```python
from build123d import *

# Parameters (mm, degrees)
SKETCH2_R               = 1.5
BOSS_EXTRUDE1_DEPTH     = 8
CUT_EXTRUDE1_DEPTH      = 18
CUT_EXTRUDE1_DEPTH_BACK = 18
CUT_EXTRUDE2_DEPTH      = 5
CUT_EXTRUDE3_DEPTH      = 1.5


with BuildPart() as part:
    # Sketch2 → Boss-Extrude1 (new body)
    with BuildSketch(Plane.XY):
        with BuildLine():
            Line((-3.5, 5), (3.5, 5))
            ThreePointArc((3.5, 5), (8.5, 0), (3.5, -5))
            Line((3.5, -5), (-3.5, -5))
            ThreePointArc((-3.5, -5), (-8.5, 0), (-3.5, 5))
        make_face()
        with Locations((-3.5, 0)):
            Circle(SKETCH2_R, mode=Mode.SUBTRACT)
    extrude(amount=BOSS_EXTRUDE1_DEPTH)

    # Sketch3 → Cut-Extrude1 (cut, two sides)
    with BuildSketch(Plane(origin=(0, 0, 0), x_dir=(0, 0, -1), z_dir=(1, 0, 0))) as cut_extrude1_sk:
        Polygon((-8, -2), (-4.5, -2), (-4.5, 2), (-6, 2), (-6, 5), (-8, 5), align=None)
    extrude(amount=CUT_EXTRUDE1_DEPTH, mode=Mode.SUBTRACT)
    extrude(cut_extrude1_sk.sketch, amount=-CUT_EXTRUDE1_DEPTH_BACK, mode=Mode.SUBTRACT)

    # Sketch4 → Cut-Extrude2 (cut)
    with BuildSketch(Plane.XY.offset(8)):
        with BuildLine():
            Line((-1.263932023, -2), (2.736067977, 5))
            Line((2.736067977, 5), (-10.787192153, 5))
            Line((-10.787192153, 5), (-10.787192153, -2))
            Line((-10.787192153, -2), (-5.736067977, -2))
            ThreePointArc((-5.736067977, -2), (-3.5, -3), (-1.263932023, -2))
        make_face()
    extrude(amount=-CUT_EXTRUDE2_DEPTH, mode=Mode.SUBTRACT)

    # Sketch5 → Cut-Extrude3 (cut)
    with BuildSketch(Plane.XY.offset(3)):
        Polygon((1.021782263, 2), (2.736067977, 5), (-9.199414094, 5), (-9.199414094, 2), align=None)
    extrude(amount=-CUT_EXTRUDE3_DEPTH, mode=Mode.SUBTRACT)


solid = part.part
```
Here's how the part is built. I have some questions about the finished solid (model axes, mm). A direction names the side the tool comes from. Coordinates: 2 decimals unless noted, no trailing zeros. Loops run counter-clockwise (first coordinate to the right, second up) from the corner with the lowest first, then second, coordinate; pieces in that order, holes last. Notation, with made-up numbers: (67.5, -2) -> (120.5, -2) arc R21 ccw to (120.5, 18) -> close; hole circle Ø6 at (63.25, -18.5). An arc over 180 degrees is marked (long way). Return JSON: item names as keys, results as strings.
1) For faces 4 (the face through (-3, 4, 1.5)), 5 (the face through (-3.5, -3, 5.5)), 6 (the face through (5, 3, 6)), 7 (the face through (5, 0, 4.5)), which set-ups out of +Z, -Z, +X, -X, +Y, -Y let a thin tool reach every point of the face, with its end or its side?
Results below:
{"face 4": "+Z, -X, +Y", "face 5": "+Z, +Y", "face 6": "+Z, +X, -X, +Y", "face 7": "+Z, +X, -X"}
2) If we section it at D-D, the plane z = 6.75: Write out the boundary of the cut face in (x, y).
Results below:
{"outline": "(-8.08, -2) arc R5 ccw to (-3.5, -5) -> (3.5, -5) arc R5 ccw to (8.08, -2) -> (-1.26, -2) arc R3 cw to (-5.74, -2) -> close"}
3) Will these pins go through, and if not, where does the flat tip stop? pin 1 (1.2 mm diameter, centred on x = -7, z = 5.5, fed in from +Y); pin 2 (4 mm diameter, centred on x = -3.5, y = 0, fed in from +Z); pin 3 (2 mm diameter, centred on x = 4, y = 0, fed in from +Z).
Results below:
{"pin 1": "y = -2", "pin 2": "z = 3", "pin 3": "z = 4.5"}
4) Thinking about a two-plate mould opening in X: for faces 1 (the face through (0, -5, 4)), 2 (the face through (-5, 1, 3)), 3 (the face through (-7.259, -3.297, 3.055)), which applies, +X half, -X half, draft (parallel to the pull), parting line (faces both ways), or undercut?
Results below:
{"face 1": "draft", "face 2": "undercut", "face 3": "-X half"}
5) If we section it at A-A, the plane z = 3.25: Write out the boundary of the cut face in (x, y).
Results below:
{"outline": "(-8.08, -2) arc R5 ccw to (-3.5, -5) -> (3.5, -5) arc R5 ccw to (3.5, 5) -> (2.74, 5) -> (-1.26, -2) arc R3 cw to (-5.74, -2) -> close"}
6) If we section it at B-B, the plane y = 0: Write out the boundary of the cut face in (x, z).
Results below:
{"outline": "(-8.5, 0) -> (-5, 0) -> (-5, 3) -> (-8.5, 3) -> close; (-2, 0) -> (8.5, 0) -> (8.5, 4.5) -> (-0.12, 4.5) -> (-0.12, 3) -> (-2, 3) -> close"}
7) If we section it at C-C, the plane x = 7.5: Write out the boundary of the cut face in (y, z), then the cut area to 3 significant figures.
Results below:
{"outline": "(-3, 0) -> (3, 0) -> (3, 6) -> (2, 6) -> (2, 4.5) -> (-2, 4.5) -> (-2, 8) -> (-3, 8) -> close", "area": "32.0 mm²"}
8) I need wall thicknesses on line 1 (Y direction, x = -3.5, z = 0.95); line 2 (X direction, y = 0, z = 2.3); line 3 (Z direction, x = -6.5, y = 1.75). Which ranges of each line are inside material? Lowest first, please. Write a range as from..to.
Results below:
{"line 1": "-5..-1.5, 1.5..5", "line 2": "-8.5..-5, -2..8.5", "line 3": "0..3"}
